Here's how the part is built. I have some questions about the finished solid (model axes, mm). Coordinates: 2 decimals unless noted, no trailing zeros. Loops run counter-clockwise (first coordinate to the right, second up) from the corner with the lowest first, then second, coordinate; pieces in that order, holes last.
from build123d import *

# Parameters (mm, degrees)
SKETCH_1_W          = 100
SKETCH_1_H          = 10
EXTRUDE_1_DEPTH     = 1.5
SKETCH_2_R          = 1.5
CUT_EXTRUDE_1_DEPTH = 10
FILLET_1_R          = 2


with BuildPart() as part:
    # 草图1 → 凸台-拉伸1 (new, symmetric)
    with BuildSketch(Plane.XY):
        Rectangle(SKETCH_1_W, SKETCH_1_H)
    extrude(amount=EXTRUDE_1_DEPTH, both=True)

    # 草图2 → 切除-拉伸1 (cut)
    with BuildSketch(Plane.XY.offset(1.5)):
        with Locations((-45, 0)):
            Circle(SKETCH_2_R)
        with Locations((45, 0)):
            Circle(SKETCH_2_R)
    extrude(amount=-CUT_EXTRUDE_1_DEPTH, mode=Mode.SUBTRACT)

    # 圆角1
    fillet_1_edges = [part.edges().sort_by_distance(p)[0] for p in [
        (0, -5, -1.5),
        (-50, 0, -1.5),
        (0, 5, -1.5),
        (50, 0, -1.5),
        (50, -5, 0),
        (-50, -5, 0),
        (-50, 5, 0),
        (50, 5, 0),
    ]]
    fillet(fillet_1_edges, radius=FILLET_1_R)


solid = part.part
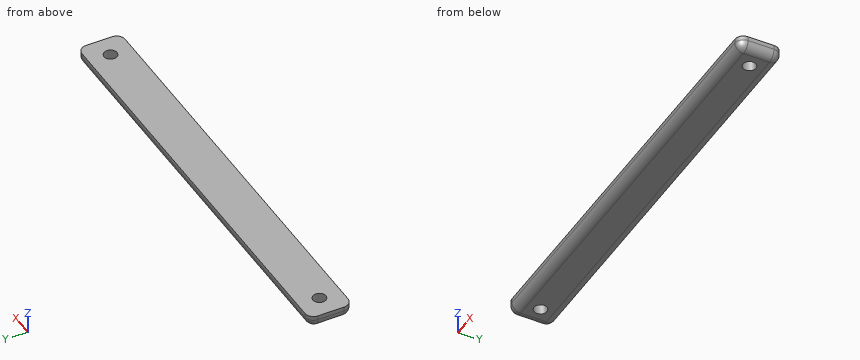
Q1. Please list where these lines run through material, in increasing order: probe 1 along Y at (x, z) = (-45, 0.8); probe 2 along X at (y, z) = (1.25, -1.2); probe 3 along Y at (x, z) = (-45, -0.65).
Q2. Suppose I cut it at B-B on y = 0. Write out the boundary of the cut face in (x, z), and give its area (3 significant figures).
Q3. Suppose I cut it at D-D on x = 1. Write out the boundary of the cut face in (y, z).
Q4. Suppose I cut it at A-A on x = -45. Write out the boundary of the cut face in (y, z).
Q5. Suppose I cut it at C-C on z = -0.95. Write out the boundary of the cut face in (x, y) (1 decimal).
Q6. Will these pins go through, and if not, where does the flat tip stop? P1, Ø2.5, axis at x = -45, y = 0, coming from the -Z side; P2, Ø4, axis at x = 45, y = 0, coming from the +Z side.
Check values:
1. probe 1: y = -5 to -1.5, 1.5 to 5
1. probe 2: x = -49.05 to -45.83, -44.17 to 44.17, 45.83 to 49.05
1. probe 3: y = -4.64 to -1.5, 1.5 to 4.64
2. outline: (-50, 0.5) arc R2 ccw to (-48, -1.5) - (-46.5, -1.5) - (-46.5, 1.5) - (-50, 1.5) - close; (-43.5, -1.5) - (43.5, -1.5) - (43.5, 1.5) - (-43.5, 1.5) - close; (46.5, -1.5) - (48, -1.5) arc R2 ccw to (50, 0.5) - (50, 1.5) - (46.5, 1.5) - close
2. area: 280 mm2
3. outline: (-5, 0.5) arc R2 ccw to (-3, -1.5) - (3, -1.5) arc R2 ccw to (5, 0.5) - (5, 1.5) - (-5, 1.5) - close
4. outline: (-5, 0.5) arc R2 ccw to (-3, -1.5) - (-1.5, -1.5) - (-1.5, 1.5) - (-5, 1.5) - close; (1.5, -1.5) - (3, -1.5) arc R2 ccw to (5, 0.5) - (5, 1.5) - (1.5, 1.5) - close
5. outline: (-49.4, -3) arc R1.4 ccw to (-48, -4.4) - (48, -4.4) arc R1.4 ccw to (49.4, -3) - (49.4, 3) arc R1.4 ccw to (48, 4.4) - (-48, 4.4) arc R1.4 ccw to (-49.4, 3) - close; hole circle Ø3 at (-45, 0); hole circle Ø3 at (45, 0)
6. P1: passes through
6. P2: stops at z = 1.5
